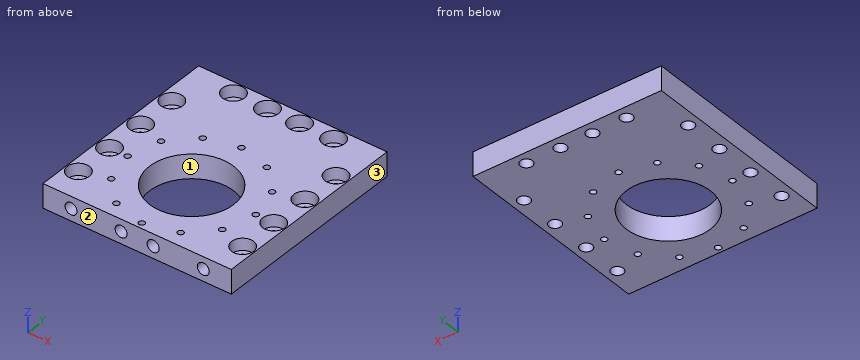
from build123d import *

# Parameters (mm, degrees)
SKETCH_1_W          = 70
SKETCH_1_H          = 70
SKETCH_1_R          = 21
SKETCH_1_R_2        = 1.5
EXTRUDE_1_DEPTH     = 12
SKETCH_3_W          = 70
SKETCH_3_H          = 12
EXTRUDE_2_DEPTH     = 30
SKETCH_4_R          = 3
CUT_EXTRUDE_2_DEPTH = 12
SKETCH_7_R          = 5.5
CUT_EXTRUDE_6_DEPTH = 6
SKETCH_8_W          = 12
SKETCH_8_H          = 100
EXTRUDE_3_DEPTH     = 12
SKETCH_11_W         = 12
SKETCH_11_H         = 100
EXTRUDE_4_DEPTH     = 12
SKETCH_12_R         = 3
CUT_EXTRUDE_7_DEPTH = 22
SKETCH_13_R         = 5.5
CUT_EXTRUDE_8_DEPTH = 6
SKETCH_14_R         = 3
CUT_EXTRUDE_9_DEPTH = 10


with BuildPart() as part:
    # 草图1 → 凸台-拉伸1 (new body)
    with BuildSketch(Plane.XY):
        Rectangle(SKETCH_1_W, SKETCH_1_H)
        Circle(SKETCH_1_R, mode=Mode.SUBTRACT)
        with Locations((32, 0)):
            Circle(SKETCH_1_R_2, mode=Mode.SUBTRACT)
        with Locations((27.712812921, -16)):
            Circle(SKETCH_1_R_2, mode=Mode.SUBTRACT)
        with Locations((16, -27.712812921)):
            Circle(SKETCH_1_R_2, mode=Mode.SUBTRACT)
        with Locations((0, -32)):
            Circle(SKETCH_1_R_2, mode=Mode.SUBTRACT)
        with Locations((-16, -27.712812921)):
            Circle(SKETCH_1_R_2, mode=Mode.SUBTRACT)
        with Locations((-27.712812921, -16)):
            Circle(SKETCH_1_R_2, mode=Mode.SUBTRACT)
        with Locations((-32, 0)):
            Circle(SKETCH_1_R_2, mode=Mode.SUBTRACT)
        with Locations((-27.712812921, 16)):
            Circle(SKETCH_1_R_2, mode=Mode.SUBTRACT)
        with Locations((-16, 27.712812921)):
            Circle(SKETCH_1_R_2, mode=Mode.SUBTRACT)
        with Locations((0, 32)):
            Circle(SKETCH_1_R_2, mode=Mode.SUBTRACT)
        with Locations((16, 27.712812921)):
            Circle(SKETCH_1_R_2, mode=Mode.SUBTRACT)
        with Locations((27.712812921, 16)):
            Circle(SKETCH_1_R_2, mode=Mode.SUBTRACT)
    extrude(amount=EXTRUDE_1_DEPTH)

    # 草图3 → 凸台-拉伸2 (add)
    with BuildSketch(Plane(origin=(0, 35, 0), x_dir=(1, 0, 0), z_dir=(0, 1, 0))):
        with Locations((0, -6)):
            Rectangle(SKETCH_3_W, SKETCH_3_H)
    extrude(amount=EXTRUDE_2_DEPTH)

    # 草图4 → 切除-拉伸2 (cut)
    with BuildSketch(Plane(origin=(0, 0, 0), x_dir=(-1, 0, 0), z_dir=(0, 0, -1))):
        with Locations((-25, 59)):
            Circle(SKETCH_4_R)
        with Locations((-8, 59)):
            Circle(SKETCH_4_R)
        with Locations(Location((25, 59, 0), (0, 0, 180))):
            Circle(SKETCH_4_R)
        with Locations(Location((8, 59, 0), (0, 0, 180))):
            Circle(SKETCH_4_R)
    extrude(amount=-CUT_EXTRUDE_2_DEPTH, mode=Mode.SUBTRACT)

    # 草图7 → 切除-拉伸6 (cut)
    with BuildSketch(Plane.XY.offset(12)):
        with Locations((-25, 59)):
            Circle(SKETCH_7_R)
        with Locations((-8, 59)):
            Circle(SKETCH_7_R)
        with Locations((8, 59)):
            Circle(SKETCH_7_R)
        with Locations((25, 59)):
            Circle(SKETCH_7_R)
    extrude(amount=-CUT_EXTRUDE_6_DEPTH, mode=Mode.SUBTRACT)

    # 草图8 → 凸台-拉伸3 (add)
    with BuildSketch(Plane(origin=(35, 0, 0), x_dir=(0, 0, -1), z_dir=(1, 0, 0))):
        with Locations((-6, 15)):
            Rectangle(SKETCH_8_W, SKETCH_8_H)
    extrude(amount=EXTRUDE_3_DEPTH)

    # 草图11 → 凸台-拉伸4 (add)
    with BuildSketch(Plane.ZY.offset(35)):
        with Locations((6, 15)):
            Rectangle(SKETCH_11_W, SKETCH_11_H)
    extrude(amount=EXTRUDE_4_DEPTH)

    # 草图12 → 切除-拉伸7 (cut)
    with BuildSketch(Plane.XY.offset(12)):
        with Locations((41, -20)):
            Circle(SKETCH_12_R)
        with Locations((41, 0)):
            Circle(SKETCH_12_R)
        with Locations((41, 20)):
            Circle(SKETCH_12_R)
        with Locations((41, 40)):
            Circle(SKETCH_12_R)
        with Locations((-41, -20)):
            Circle(SKETCH_12_R)
        with Locations((-41, 0)):
            Circle(SKETCH_12_R)
        with Locations((-41, 40)):
            Circle(SKETCH_12_R)
        with Locations((-41, 20)):
            Circle(SKETCH_12_R)
    extrude(amount=-CUT_EXTRUDE_7_DEPTH, mode=Mode.SUBTRACT)

    # 草图13 → 切除-拉伸8 (cut)
    with BuildSketch(Plane.XY.offset(12)):
        with Locations((41, 40)):
            Circle(SKETCH_13_R)
        with Locations((41, 20)):
            Circle(SKETCH_13_R)
        with Locations((41, 0)):
            Circle(SKETCH_13_R)
        with Locations(Location((-41, -20, 0), (0, 0, 180))):
            Circle(SKETCH_13_R)
        with Locations((41, -20)):
            Circle(SKETCH_13_R)
        with Locations(Location((-41, 0, 0), (0, 0, 180))):
            Circle(SKETCH_13_R)
        with Locations(Location((-41, 20, 0), (0, 0, 180))):
            Circle(SKETCH_13_R)
        with Locations(Location((-41, 40, 0), (0, 0, 180))):
            Circle(SKETCH_13_R)
    extrude(amount=-CUT_EXTRUDE_8_DEPTH, mode=Mode.SUBTRACT)

    # 草图14 → 切除-拉伸9 (cut)
    with BuildSketch(Plane.XZ.offset(35)):
        with Locations(Location((-33, 6, 0), (0, 0, 270))):
            Circle(SKETCH_14_R)
        with Locations(Location((-8, 6, 0), (0, 0, 270))):
            Circle(SKETCH_14_R)
        with Locations(Location((33, 6, 0), (0, 0, 90))):
            Circle(SKETCH_14_R)
        with Locations(Location((8, 6, 0), (0, 0, 90))):
            Circle(SKETCH_14_R)
    extrude(amount=-CUT_EXTRUDE_9_DEPTH, mode=Mode.SUBTRACT)


solid = part.part
Can you work these out from the model? Positions are in its coordinate system, mm. Face numbers are marked on the shaded views. Give positions to 0.01 mm unless a question says otherwise; leave off trailing zeros. Loops run counter-clockwise (first coordinate to the right, second up) from the corner with the lowest first, then second, coordinate; pieces in that order, holes last. Notation, with made-up numbers: (-19, -38) -> (5, -38) arc R30 ccw to (5, 0) -> close; hole circle Ø7 at (88.5, -14). An arc over 180 degrees is marked (long way). Return JSON: item names as keys, results as strings.
Q1. We'd pull the mould along X, two halves only. Please class the marked faces 1, 2 and 3: released by +X, released by -X, zero draft, split by the parting line, or undercut.
Checks:
{"face 1": "undercut", "face 2": "zero draft", "face 3": "released by +X"}
Q2. I want a section at A-A, the plane y = 0. Count the separate pieces of the cut face and the enclosed holes in it, then the cut area to 3 significant figures.
Checks:
{"separate pieces": "6", "enclosed holes": "0", "area": "348 mm2"}
Q3. I need wall thicknesses on probe 1 along Y at (x, z) = (41, 9); probe 2 along X at (y, z) = (37.5, 10.25); probe 3 along X at (y, z) = (38, 1). Which ranges of each line are inside material? Lowest first, please.
Checks:
{"probe 1": "y = -35 to -25.5, -14.5 to -5.5, 5.5 to 14.5, 25.5 to 34.5, 45.5 to 65", "probe 2": "x = -47 to -45.9, -36.1 to 36.1, 45.9 to 47", "probe 3": "x = -47 to -43.24, -38.76 to 38.76, 43.24 to 47"}
Q4. I want a section at C-C, the plane x = -25. List the corners of the cut face in (y, z) for me.
Checks:
{"outline": "(-35, 0) -> (56, 0) -> (56, 6) -> (53.5, 6) -> (53.5, 12) -> (-35, 12) -> close; (62, 0) -> (65, 0) -> (65, 12) -> (64.5, 12) -> (64.5, 6) -> (62, 6) -> close"}
Q5. For pin 1 Ø3.5 at (x, y) = (39.5, -18) entering from +Z; pin 2 Ø2.5 at (x, y) = (-32, 0) entering from -Z, each with a flat end and sliding along its axis, tell me the tip position at first contact or that it passes through.
Checks:
{"pin 1": "stops at z = 6", "pin 2": "passes through"}
Q6. I want a section at B-B, the plane y = 32. List the corners of the cut face in (x, z) for me.
Checks:
{"outline": "(-47, 0) -> (-1.5, 0) -> (-1.5, 12) -> (-47, 12) -> close; (1.5, 0) -> (47, 0) -> (47, 12) -> (1.5, 12) -> close"}
